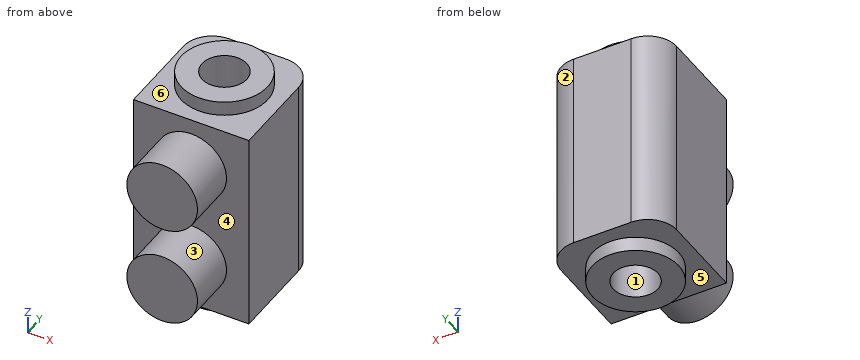
```python
from build123d import *

# Parameters (mm, degrees)
SKETCH1_W           = 8
SKETCH1_H           = 14
BOSS_EXTRUDE1_DEPTH = 8
SKETCH2_R           = 2.45
BOSS_EXTRUDE2_DEPTH = 3.5
FILLET1_R           = 2
SKETCH5_R           = 3
BOSS_EXTRUDE3_DEPTH = 1
SKETCH6_R           = 1.55
CUT_EXTRUDE1_DEPTH  = 20.595917942


with BuildPart() as part:
    # Sketch1 → Boss-Extrude1 (new body)
    with BuildSketch(Plane(origin=(0, 0, 0), x_dir=(1, 0, 0), z_dir=(0, 1, 0))):
        with Locations((4, 7)):
            Rectangle(SKETCH1_W, SKETCH1_H)
    extrude(amount=BOSS_EXTRUDE1_DEPTH)

    # Sketch2 → Boss-Extrude2 (add)
    with BuildSketch(Plane.XZ):
        with Locations(Location((4, -10.5, 0), (0, 0, 270))):
            Circle(SKETCH2_R)
        with Locations(Location((4, -3.5, 0), (0, 0, 90))):
            Circle(SKETCH2_R)
    extrude(amount=BOSS_EXTRUDE2_DEPTH)

    # Fillet1
    fillet1_edges = [part.edges().sort_by_distance(p)[0] for p in [
        (8, 8, -7),
        (0, 8, -7),
    ]]
    fillet(fillet1_edges, radius=FILLET1_R)

    # Sketch5 → Boss-Extrude3 (add)
    with BuildSketch(Plane(origin=(0, 0, -14), x_dir=(-1, 0, 0), z_dir=(0, 0, -1))):
        with Locations((-4, 4)):
            Circle(SKETCH5_R)
    boss_extrude3 = extrude(amount=BOSS_EXTRUDE3_DEPTH)

    # Mirror1: Boss-Extrude3 across plane
    add(boss_extrude3.mirror(Plane(origin=(0, 0, -7), x_dir=(1, 0, 0), z_dir=(0, 0, -1))))

    # Sketch6 → Cut-Extrude1 (cut, through all)
    with BuildSketch(Plane(origin=(0, 0, -15), x_dir=(-1, 0, 0), z_dir=(0, 0, -1))):
        with Locations((-4, 4)):
            Circle(SKETCH6_R)
    extrude(amount=-CUT_EXTRUDE1_DEPTH, mode=Mode.SUBTRACT)


solid = part.part
```
Check sheet for the modelled part. Datum: model origin and axes. Units: mm. Face numbers are marked on the shaded views. A direction names the side the tool comes from. Coordinates: 2 decimals unless noted, no trailing zeros. Loops run counter-clockwise (first coordinate to the right, second up) from the corner with the lowest first, then second, coordinate; pieces in that order, holes last.
1) Sectioned sample at B-B (z = -3.5). Record the boundary of the cut face in (x, y).
2) Sectioned sample at A-A (y = 4). Record the boundary of the cut face in (x, z).
3) Material ranges on probe 1 along Y at (x, z) = (4, -6.25); probe 2 along Y at (x, z) = (4, -3.25); probe 3 along Z at (x, y) = (7.5, 0.5), recorded low to high.
4) Release check for a two-part mould opening along Y. For the marked faces 1, 2 and 3 record: released by +Y, released by -Y, zero draft, split by the parting line, or undercut.
5) Sectioned sample at C-C (x = 4). Record the boundary of the cut face in (y, z), and give its area (3 significant figures).
6) Gauge pin test, flat end, axial feed: pin 1 (1.5 mm diameter, centred on x = 6.5, y = 7, fed in from -Z). Record the tip position at first contact, or that the pin passes through.
7) Sectioned sample at D-D (z = -7). Record the boundary of the cut face in (x, y), and give its area (3 significant figures).
8) Access from +Z, -Z, +X, -X, +Y, -Y to the whole of each face (thin tool, end or side, straight path). Record for the marked faces 4, 5 and 6.
Check sheet entries:
1. outline: (0, 0) - (1.55, 0) - (1.55, -3.5) - (6.45, -3.5) - (6.45, 0) - (8, 0) - (8, 6) arc R2 ccw to (6, 8) - (2, 8) arc R2 ccw to (0, 6) - close; hole circle Ø3.1 at (4, 4)
2. outline: (0, -14) - (1, -14) - (1, -15) - (2.45, -15) - (2.45, 1) - (1, 1) - (1, 0) - (0, 0) - close; (5.55, -15) - (7, -15) - (7, -14) - (8, -14) - (8, 0) - (7, 0) - (7, 1) - (5.55, 1) - close
3. probe 1: y = 0 to 2.45, 5.55 to 8
3. probe 2: y = -3.5 to 2.45, 5.55 to 8
3. probe 3: z = -14 to 0
4. face 1: undercut
4. face 2: released by +Y
4. face 3: zero draft
5. outline: (-3.5, -12.95) - (0, -12.95) - (0, -14) - (1, -14) - (1, -15) - (2.45, -15) - (2.45, 1) - (1, 1) - (1, 0) - (0, 0) - (0, -1.05) - (-3.5, -1.05) - (-3.5, -5.95) - (0, -5.95) - (0, -8.05) - (-3.5, -8.05) - close; (5.55, -15) - (7, -15) - (7, -14) - (8, -14) - (8, 0) - (7, 0) - (7, 1) - (5.55, 1) - close
5. area: 109 mm2
6. pin 1: stops at z = -14
7. outline: (0, 0) - (8, 0) - (8, 6) arc R2 ccw to (6, 8) - (2, 8) arc R2 ccw to (0, 6) - close; hole circle Ø3.1 at (4, 4)
7. area: 54.7 mm2
8. face 4: -Y
8. face 5: -Z
8. face 6: +Z
